Build history of the part. All positions in model axes, mm. A direction names the side the tool comes from. Give positions to 0.01 mm unless a question says otherwise; leave off trailing zeros. Loops run counter-clockwise (first coordinate to the right, second up) from the corner with the lowest first, then second, coordinate; pieces in that order, holes last. Notation, with made-up numbers: M -11,6 L 35,6 A21 cw 35,35 Z; hole C -12.75,26 d2. An arc over 180 degrees is marked long. Put each result on its own line as item: value.
```python
from build123d import *

# Parameters (mm, degrees)
EXTRUDE_START          = -1.5
SKETCH_1_R             = 12.5
EXTRUDE_1_DEPTH        = 227.9
HOLE_WIZARD_M101_D     = 8.5
HOLE_WIZARD_M101_DEPTH = 30
HOLE_WIZARD_M101_TIP   = 2.553657631
HOLE_WIZARD_M102_D     = 8.5
HOLE_WIZARD_M102_DEPTH = 32.5
HOLE_WIZARD_M102_TIP   = 2.553657631
SKETCH_6_W             = 8
SKETCH_6_H             = 8
CUT_EXTRUDE_1_DEPTH    = 30


with BuildPart() as part:
    # Эскиз1 → Бобышка-Вытянуть1 (new body)
    with BuildSketch(Plane.XY.offset(EXTRUDE_START)):
        with Locations((0.192463074, -155.807573628)):
            Circle(SKETCH_1_R)
    extrude(amount=-EXTRUDE_1_DEPTH)

    # Отверстие обработанное метчиком M101
    with Locations(Plane.XY.offset(-1.5)):
        with Locations((0.192463074, -155.807573628)):
            Hole(HOLE_WIZARD_M101_D / 2, depth=HOLE_WIZARD_M101_DEPTH)
            with Locations((0, 0, -(HOLE_WIZARD_M101_DEPTH + HOLE_WIZARD_M101_TIP / 2))):  # 118° drill point
                Cone(0, HOLE_WIZARD_M101_D / 2, HOLE_WIZARD_M101_TIP, mode=Mode.SUBTRACT)

    # Отверстие обработанное метчиком M102
    with Locations(Plane(origin=(0, 0, -229.4), x_dir=(-1, 0, 0), z_dir=(0, 0, -1))):
        with Locations((-0.192463074, -155.807573628)):
            Hole(HOLE_WIZARD_M102_D / 2, depth=HOLE_WIZARD_M102_DEPTH)
            with Locations((0, 0, -(HOLE_WIZARD_M102_DEPTH + HOLE_WIZARD_M102_TIP / 2))):  # 118° drill point
                Cone(0, HOLE_WIZARD_M102_D / 2, HOLE_WIZARD_M102_TIP, mode=Mode.SUBTRACT)

    # Эскиз6 → Вырез-Вытянуть1 (cut)
    with BuildSketch(Plane.XY.offset(-1.5)):
        with Locations((-12.307536926, -155.807573628)):
            Rectangle(SKETCH_6_W, SKETCH_6_H)
    extrude(amount=-CUT_EXTRUDE_1_DEPTH, mode=Mode.SUBTRACT)


solid = part.part
```
Q1. Mould opens along Y. For faces 1 (the flat face through (6, -156, -1.5)), 2 (the cylindrical face through (11.739, -160.595, -113.855)), 3 (the flat face through (-10, -156, -31.5)), 4 (the conical face through (-0.204, -155.185, -194.79)) say: pulls with the +Y half, pulls with the -Y half, needs draft (parallel to the pull), parting line crosses it, or undercut.
Here are the results:
face 1: needs draft
face 2: parting line crosses it
face 3: undercut
face 4: undercut
Q2. Probe line 1 (X direction, y = -154.75, z = -72); line 2 (Y direction, x = 0.5, z = -153); line 3 (X direction, y = -156, z = -113.5). List the from-to ranges inside material, lowest first. Write a range as from..to.
Here are the results:
line 1: -12.26..12.65
line 2: -168.3..-143.31
line 3: -12.31..12.69
Q3. Slice it at D-D (z = -114). List the corners of the cut face in (x, y), and give its area (3 significant figures).
Here are the results:
outline: C 0.19,-155.81 d25
area: 491 mm²
Q4. Drop flat-ended pins along their axis: pin 1 Ø1.7 at (x, z) = (-10.5, -17.5) entering from +Y; pin 2 Ø7 at (x, y) = (0.19, -155.81) entering from +Z; pin 3 Ø8 at (y, z) = (-153, -29.5) entering from +X; pin 4 Ø2.5 at (x, z) = (-10.5, -15.5) entering from -Y. Give the stop position or say it passes through.
Here are the results:
pin 1: y = -148.1
pin 2: z = -31.95
pin 3: x = 12.69
pin 4: y = -164
Q5. Slice it at A-A (z = -28.5). List the corners of the cut face in (x, y), and give its area (3 significant figures).
Here are the results:
outline: M -11.65,-159.81 A12.5 ccw long -11.65,-151.81 L -8.31,-151.81 L -8.31,-159.81 Z; hole C 0.19,-155.81 d8.5
area: 404 mm²
Q6. Slice it at B-B (y = -148.5). List the corners of the cut face in (x, z), and give its area (3 significant figures).
Here are the results:
outline: M -9.95,-229.4 L 10.33,-229.4 L 10.33,-1.5 L -9.95,-1.5 Z
area: 4,620 mm²
Q7. Slice it at C-C (x = 9). List the corners of the cut face in (y, z).
Here are the results:
outline: M -164.68,-229.4 L -146.94,-229.4 L -146.94,-1.5 L -164.68,-1.5 Z
Q8. Tool access for faces 5 (the cylindrical face through (-0.4, -151.6, -212.9)), 6 (the flat face through (6, -156, -229.4)), 7 (the cylindrical face through (0.746, -151.594, -16.71)), 8 (the flat face through (-8.308, -156, -16)): list every direction of +Z, -Z, +X, -X, +Y, -Y with a clear straight run to the whole face (end or side of a thin tool).
Here are the results:
face 5: -Z
face 6: -Z, +X, -X, +Y, -Y
face 7: +Z
face 8: +Z, -X
